Verification items for this drawing (mm, ordinates from the low corner). A direction names the side the tool comes from. Round coordinates to 2 decimals unless told otherwise and drop trailing zeros. Write each loop counter-clockwise with the first axis right and the second up, starting at its lowest first coordinate (ties: lowest second). Pieces come first, ordered by that corner, then holes. Notation, with made-up numbers: (22.5, 59.25) -> (32.5, 59.25) arc R14 cw to (32.5, 83.25) -> close; hole circle Ø11 at (74.5, 13.5). An arc over 180 degrees is marked (long way). Use one line per item in the form item = value. Start each with the question number.
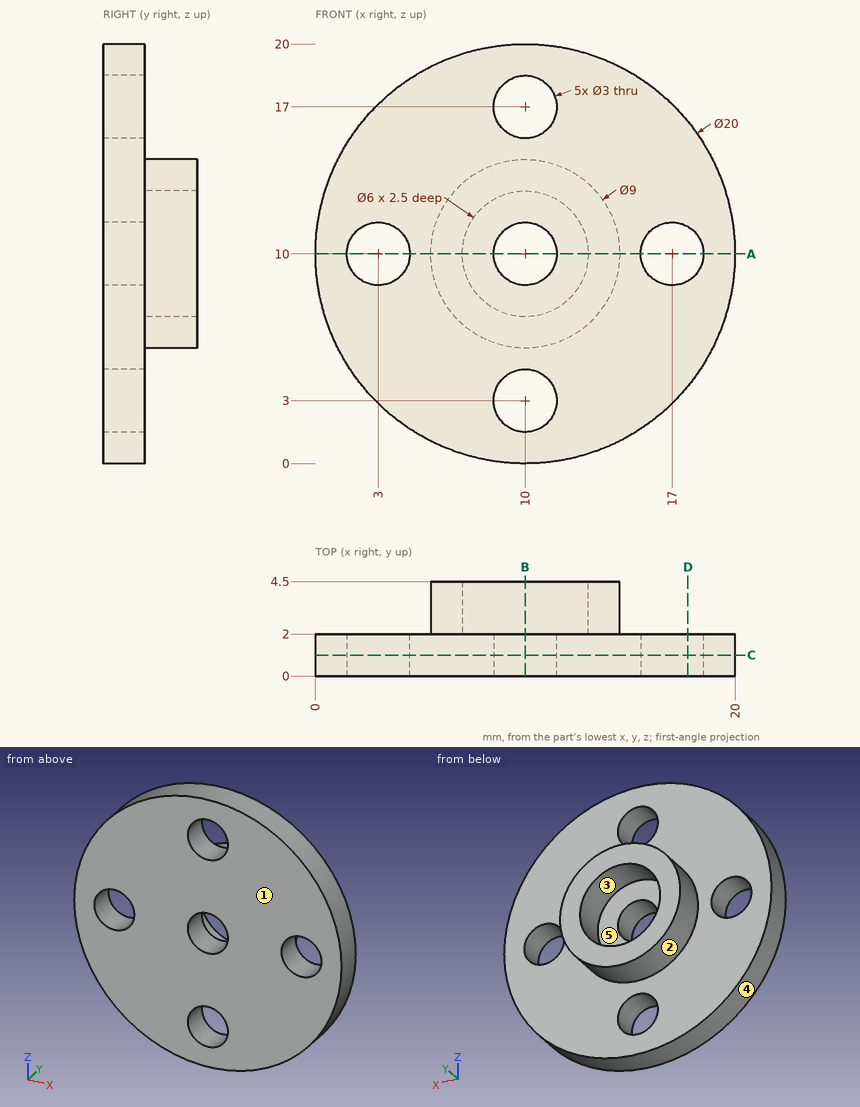
1. Sectioned sample at A-A (z = 10). Enter the section's corners in (x, y).
2. Depth check by flat-ended pin: pin 1 (1.8 mm diameter, centred on x = 3, z = 10, fed in from -Y); pin 2 (1.8 mm diameter, centred on x = 9.5, z = 9, fed in from +Y); pin 3 (2 mm diameter, centred on y = 2, z = 6, fed in from -X); pin 4 (2 mm diameter, centred on y = 3.5, z = 13, fed in from +X). Enter the tip coordinate at first touch or a pass-through.
3. Mould release check, pull along X, two halves, no side actions. Record for the marked faces 1, 2 and 3: +X half, -X half, draft (parallel to the pull), parting line (faces both ways), or undercut.
4. Tool access check on the marked faces 4 and 5. Record the directions out of +Z, -Z, +X, -X, +Y, -Y that give a thin tool (end or side, any length) a straight path to the whole face; none if there is none.
5. Sectioned sample at B-B (x = 10). Enter the section's corners in (y, z), and give its area (3 significant figures).
6. Scan lines: probe 1 along Z at (x, y) = (10, 1.65); probe 2 along Y at (x, z) = (15, 3.5). Record each from-to range of solid material in increasing order.
7. Sectioned sample at D-D (x = 17.75). Enter the section's corners in (y, z), and give its area (3 significant figures).
8. Sectioned sample at C-C (y = 1). Enter the section's corners in (x, z).
Returned:
q1.outline = (0, 0) -> (1.5, 0) -> (1.5, 2) -> (0, 2) -> close; (4.5, 0) -> (8.5, 0) -> (8.5, 2) -> (7, 2) -> (7, 4.5) -> (5.5, 4.5) -> (5.5, 2) -> (4.5, 2) -> close; (11.5, 0) -> (15.5, 0) -> (15.5, 2) -> (14.5, 2) -> (14.5, 4.5) -> (13, 4.5) -> (13, 2) -> (11.5, 2) -> close; (18.5, 0) -> (20, 0) -> (20, 2) -> (18.5, 2) -> close
q2.pin_1 = through
q2.pin_2 = 2
q2.pin_3 = 0.46
q2.pin_4 = 14.03
q3.face_1 = draft
q3.face_2 = parting line
q3.face_3 = undercut
q4.face_4 = +Y, -Y
q4.face_5 = +Y
q5.outline = (0, 0) -> (2, 0) -> (2, 1.5) -> (0, 1.5) -> close; (0, 4.5) -> (2, 4.5) -> (2, 5.5) -> (4.5, 5.5) -> (4.5, 7) -> (2, 7) -> (2, 8.5) -> (0, 8.5) -> close; (0, 11.5) -> (2, 11.5) -> (2, 13) -> (4.5, 13) -> (4.5, 14.5) -> (2, 14.5) -> (2, 15.5) -> (0, 15.5) -> close; (0, 18.5) -> (2, 18.5) -> (2, 20) -> (0, 20) -> close
q5.area = 29.5 mm^2
q6.probe_1 = 0 to 1.5, 4.5 to 8.5, 11.5 to 15.5, 18.5 to 20
q6.probe_2 = 0 to 2
q7.outline = (0, 3.68) -> (2, 3.68) -> (2, 8.7) -> (0, 8.7) -> close; (0, 11.3) -> (2, 11.3) -> (2, 16.32) -> (0, 16.32) -> close
q7.area = 20.1 mm^2
q8.outline = circle Ø20 at (10, 10); hole circle Ø3 at (3, 10); hole circle Ø3 at (10, 3); hole circle Ø3 at (10, 10); hole circle Ø3 at (10, 17); hole circle Ø3 at (17, 10)
